```python
from build123d import *

# Parameters (mm, degrees)
BOSS_EXTRUDE1_DEPTH = 150
SKETCH2_W           = 10
SKETCH2_H           = 7
BOSS_EXTRUDE4_DEPTH = 50
SKETCH4_R           = 1
CUT_EXTRUDE2_DEPTH  = 50
SKETCH5_W           = 10
SKETCH5_H           = 7
CUT_EXTRUDE3_DEPTH  = 50
SKETCH6_R           = 1
CUT_EXTRUDE4_DEPTH  = 100


with BuildPart() as part:
    # Sketch1 → Boss-Extrude1 (new body)
    with BuildSketch(Plane.XY):
        with BuildLine():
            Line((-15, 12.912739296), (15, 12.912739296))
            Line((15, 12.912739296), (15, 15.412739296))
            Line((15, 15.412739296), (11.5, 15.412739296))
            ThreePointArc((11.5, 15.412739296), (11.146446609, 15.559185905), (11, 15.912739296))
            Line((11, 15.912739296), (11, 17.028604707))
            ThreePointArc((11, 17.028604707), (11.146446609, 17.382158098), (11.5, 17.528604707))
            Line((11.5, 17.528604707), (18.5, 17.528604707))
            ThreePointArc((18.5, 17.528604707), (18.853553391, 17.382158098), (19, 17.028604707))
            Line((19, 17.028604707), (19, 10.028604707))
            ThreePointArc((19, 10.028604707), (18.853553391, 9.675051316), (18.5, 9.528604707))
            Line((18.5, 9.528604707), (15, 9.528604707))
            Line((15, 9.528604707), (15, 7.528604707))
            Line((15, 7.528604707), (18.5, 7.528604707))
            ThreePointArc((18.5, 7.528604707), (18.853553391, 7.382158098), (19, 7.028604707))
            Line((19, 7.028604707), (19, 6.028604707))
            ThreePointArc((19, 6.028604707), (18.853553391, 5.675051316), (18.5, 5.528604707))
            Line((18.5, 5.528604707), (11, 5.528604707))
            Line((11, 5.528604707), (11, 3.028604707))
            Line((11, 3.028604707), (18.661195157, 3.028604707))
            ThreePointArc((18.661195157, 3.028604707), (19.014748547, 2.882158098), (19.161195157, 2.528604707))
            Line((19.161195157, 2.528604707), (19.161195157, 1.528604707))
            Line((19.161195157, 1.528604707), (26.029307443, 1.528604707))
            ThreePointArc((26.029307443, 1.528604707), (26.382860834, 1.382158098), (26.529307443, 1.028604707))
            Line((26.529307443, 1.028604707), (26.529307443, -0.471395293))
            Line((26.529307443, -0.471395293), (11.070535665, -0.471395293))
            Line((11.070535665, -0.471395293), (-11.070535665, -0.471395293))
            Line((-11.070535665, -0.471395293), (-26.529307443, -0.471395293))
            Line((-26.529307443, -0.471395293), (-26.529307443, 1.028604707))
            ThreePointArc((-26.529307443, 1.028604707), (-26.382860834, 1.382158098), (-26.029307443, 1.528604707))
            Line((-26.029307443, 1.528604707), (-19.161195157, 1.528604707))
            Line((-19.161195157, 1.528604707), (-19.161195157, 2.528604707))
            ThreePointArc((-19.161195157, 2.528604707), (-19.014748547, 2.882158098), (-18.661195157, 3.028604707))
            Line((-18.661195157, 3.028604707), (-11, 3.028604707))
            Line((-11, 3.028604707), (-11, 5.528604707))
            Line((-11, 5.528604707), (-18.5, 5.528604707))
            ThreePointArc((-18.5, 5.528604707), (-18.853553391, 5.675051316), (-19, 6.028604707))
            Line((-19, 6.028604707), (-19, 7.028604707))
            ThreePointArc((-19, 7.028604707), (-18.853553391, 7.382158098), (-18.5, 7.528604707))
            Line((-18.5, 7.528604707), (-15, 7.528604707))
            Line((-15, 7.528604707), (-15, 9.528604707))
            Line((-15, 9.528604707), (-18.5, 9.528604707))
            ThreePointArc((-18.5, 9.528604707), (-18.853553391, 9.675051316), (-19, 10.028604707))
            Line((-19, 10.028604707), (-19, 17.028604707))
            ThreePointArc((-19, 17.028604707), (-18.853553391, 17.382158098), (-18.5, 17.528604707))
            Line((-18.5, 17.528604707), (-11.5, 17.528604707))
            ThreePointArc((-11.5, 17.528604707), (-11.146446609, 17.382158098), (-11, 17.028604707))
            Line((-11, 17.028604707), (-11, 15.912739296))
            ThreePointArc((-11, 15.912739296), (-11.146446609, 15.559185905), (-11.5, 15.412739296))
            Line((-11.5, 15.412739296), (-15, 15.412739296))
            Line((-15, 15.412739296), (-15, 12.912739296))
        make_face()
    extrude(amount=BOSS_EXTRUDE1_DEPTH)

    # Sketch2 → Boss-Extrude4 (add)
    with BuildSketch(Plane.XY.offset(150)):
        with Locations((0, 4.412739296)):
            Rectangle(SKETCH2_W, SKETCH2_H)
    extrude(amount=BOSS_EXTRUDE4_DEPTH)

    # Sketch4 → Cut-Extrude2 (cut)
    with BuildSketch(Plane(origin=(5, 0, 0), x_dir=(0, 0, -1), z_dir=(1, 0, 0))):
        with Locations(Location((-175, 4.282739296, 0), (0, 0, 90))):
            Circle(SKETCH4_R)
    extrude(amount=-CUT_EXTRUDE2_DEPTH, mode=Mode.SUBTRACT)

    # Sketch5 → Cut-Extrude3 (cut)
    with BuildSketch(Plane(origin=(0, 0, 0), x_dir=(-1, 0, 0), z_dir=(0, 0, -1))):
        with Locations((0, 4.412739296)):
            Rectangle(SKETCH5_W, SKETCH5_H)
    extrude(amount=-CUT_EXTRUDE3_DEPTH, mode=Mode.SUBTRACT)

    # Sketch6 → Cut-Extrude4 (cut)
    with BuildSketch(Plane.ZY.offset(11)):
        with Locations(Location((25, 4.278604707, 0), (0, 0, 270))):
            Circle(SKETCH6_R)
    extrude(amount=-CUT_EXTRUDE4_DEPTH, mode=Mode.SUBTRACT)


solid = part.part
```
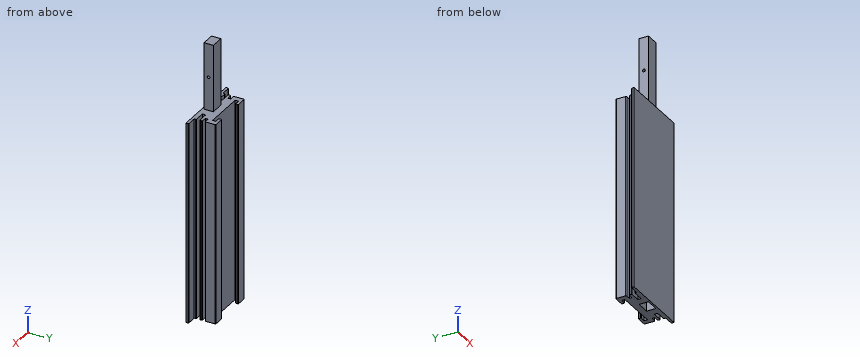
The model under review builds one solid part; all positions refer to its coordinate system, in mm. Round coordinates to 2 decimals unless told otherwise and drop trailing zeros. Order: outer loops, then holes, each group sorted by start corner. A loop starts at its lowest first (then second) coordinate and runs counter-clockwise, first axis right, second up. Notation, with made-up numbers: (1, 28) -> (8, 28) arc R12 ccw to (8, 50) -> close; hole circle Ø1 at (73, -7.5). An arc over 180 degrees is marked (long way). Use a Markdown table: item, result.
Q1. We need section A-A on x = 22. Write out the cut boundary in (y, z), then the cut area to 3 significant figures.
Values:
| item | result |
|---|---|
| outline | (-0.47, 0) -> (1.53, 0) -> (1.53, 150) -> (-0.47, 150) -> close |
| area | 300 mm^2 |
Q2. For line 1 (Y direction, x = 0, z = 175); line 2 (X direction, y = 16.25, z = 72); line 3 (Z direction, x = -12, y = 8.25), list the stretches that pass through material, from the lowest coordinate up.
Values:
| item | result |
|---|---|
| line 1 | y = 0.91 to 3.28, 5.28 to 7.91 |
| line 2 | x = -19 to -11, 11 to 19 |
| line 3 | z = 0 to 150 |
Q3. Clearance check with flat-ended pins moving along their axes: P1, Ø1, axis at x = -7, z = 132, coming from the +Y side; P2, Ø1.3, axis at y = 4, z = 68, coming from the +X side; P3, Ø5.5, axis at y = 4.5, z = 182, coming from the +X side. State where each tip first meets the part, or that it passes through.
Values:
| item | result |
|---|---|
| P1 | stops at y = 12.91 |
| P2 | stops at x = 11 |
| P3 | stops at x = 5 |
